Read the model definition and answer for the solid it produces. Units are mm, in the model's axes. A direction names the side the tool comes from. Round coordinates to 2 decimals unless told otherwise and drop trailing zeros. Order: outer loops, then holes, each group sorted by start corner. A loop starts at its lowest first (then second) coordinate and runs counter-clockwise, first axis right, second up. Notation, with made-up numbers: (41, 39) - (68, 39) arc R16 ccw to (68, 70) - close; hole circle Ø6 at (4.5, -26.5). An arc over 180 degrees is marked (long way). One line per question, with ' | ' between items. Start each with the question number.
1) Flat-ended cylindrical pins translate along their axes: pin 1 (3 mm diameter, centred on x = 20.5, y = 0, fed in from +Z); pin 2 (1.5 mm diameter, centred on x = 7.5, y = -2.5, fed in from +Z). Find the tip coordinate at first contact, or state that the pin passes through.
2) The part is cut by section C-C, the plane x = 8. Give the vertices of the cut face in (y, z), plus the area to 3 significant figures.
3) Straight lines are drawn through the part: line 1 (X direction, y = 2.25, z = -0.5); line 2 (Y direction, x = 1.5, z = -2.75); line 3 (Z direction, x = 4, y = -1.25). For each, find the intervals that lie inside material, in ascending order. Write a range as from..to.
4) For faces 1 (the cylindrical face through (22.22, 0.07, 1.5)), 2 (the cylindrical face through (10.114, -3.905, 0.867)), determine the directions among +Z, -Z, +X, -X, +Y, -Y from which every point of the face is accessible in a straight line to the end or side of a thin tool.
5) The part is cut by section A-A, the plane z = 0. Give the vertices of the cut face in (x, y).
from build123d import *

# Parameters (mm, degrees)
CROQUIS1_R              = 4
SALIENTE_EXTRUIR1_DEPTH = 20
CROQUIS2_R              = 1.5
SALIENTE_EXTRUIR2_DEPTH = 5
CHAFL_N1_SIZE           = 0.5
CHAFL_N2_SIZE           = 0.5


with BuildPart() as part:
    # Croquis1 → Saliente-Extruir1 (new body)
    with BuildSketch(Plane(origin=(0, 0, 0), x_dir=(0, 0, -1), z_dir=(1, 0, 0))):
        Circle(CROQUIS1_R)
    extrude(amount=SALIENTE_EXTRUIR1_DEPTH)

    # Croquis2 → Saliente-Extruir2 (add)
    with BuildSketch(Plane(origin=(20, 0, 0), x_dir=(0, 0, -1), z_dir=(1, 0, 0))):
        Circle(CROQUIS2_R)
    extrude(amount=SALIENTE_EXTRUIR2_DEPTH)

    # Chaflán1
    chafl_n1_edges = [part.edges().sort_by_distance(p)[0] for p in [
        (0, 0, 4),
    ]]
    chamfer(chafl_n1_edges, length=CHAFL_N1_SIZE)

    # Chaflán2
    chafl_n2_edges = [part.edges().sort_by_distance(p)[0] for p in [
        (25, 0, 1.5),
    ]]
    chamfer(chafl_n2_edges, length=CHAFL_N2_SIZE)


solid = part.part
Values:
1) pin 1: stops at z = 4 | pin 2: stops at z = 3.6
2) outline: circle Ø8 at (0, 0) | area: 50.3 mm^2
3) line 1: x = 0..20 | line 2: y = -2.9..2.9 | line 3: z = -3.8..3.8
4) face 1: +X | face 2: +X, -X
5) outline: (0, -3.5) - (0.5, -4) - (20, -4) - (20, -1.5) - (24.5, -1.5) - (25, -1) - (25, 1) - (24.5, 1.5) - (20, 1.5) - (20, 4) - (0.5, 4) - (0, 3.5) - close
